from build123d import *

# Parameters (mm, degrees)
SKETCH1_R                 = 2.5
BOSS_EXTRUDE1_DEPTH       = 30
M3X0_5_TAPPED_HOLE1_D     = 2.5
M3X0_5_TAPPED_HOLE1_DEPTH = 7
M3X0_5_TAPPED_HOLE1_TIP   = 0.751075774
M3X0_5_TAPPED_HOLE2_D     = 2.5
M3X0_5_TAPPED_HOLE2_DEPTH = 7
M3X0_5_TAPPED_HOLE2_TIP   = 0.751075774
CHAMFER1_SIZE             = 0.5


with BuildPart() as part:
    # Sketch1 → Boss-Extrude1 (new body)
    with BuildSketch(Plane(origin=(0, 0, 0), x_dir=(1, 0, 0), z_dir=(0, 1, 0))):
        with Locations(Location((0, 0, 0), (0, 0, 270))):
            Circle(SKETCH1_R)
    extrude(amount=BOSS_EXTRUDE1_DEPTH)

    # M3x0.5 Tapped Hole1
    with Locations(Plane(origin=(0, 30, 0), x_dir=(1, 0, 0), z_dir=(0, 1, 0))):
        with Locations((0, 0)):
            Hole(M3X0_5_TAPPED_HOLE1_D / 2, depth=M3X0_5_TAPPED_HOLE1_DEPTH)
            with Locations((0, 0, -(M3X0_5_TAPPED_HOLE1_DEPTH + M3X0_5_TAPPED_HOLE1_TIP / 2))):  # 118° drill point
                Cone(0, M3X0_5_TAPPED_HOLE1_D / 2, M3X0_5_TAPPED_HOLE1_TIP, mode=Mode.SUBTRACT)

    # M3x0.5 Tapped Hole2
    with Locations(Plane(origin=(0, 0, 0), x_dir=(-1, 0, 0), z_dir=(0, -1, 0))):
        with Locations((0, 0)):
            Hole(M3X0_5_TAPPED_HOLE2_D / 2, depth=M3X0_5_TAPPED_HOLE2_DEPTH)
            with Locations((0, 0, -(M3X0_5_TAPPED_HOLE2_DEPTH + M3X0_5_TAPPED_HOLE2_TIP / 2))):  # 118° drill point
                Cone(0, M3X0_5_TAPPED_HOLE2_D / 2, M3X0_5_TAPPED_HOLE2_TIP, mode=Mode.SUBTRACT)

    # Chamfer1
    chamfer1_edges = [part.edges().sort_by_distance(p)[0] for p in [
        (0, 0, -2.5),
        (0, 30, -2.5),
    ]]
    chamfer(chamfer1_edges, length=CHAMFER1_SIZE)


solid = part.part
Read the model definition and answer for the solid it produces. Units are mm, in the model's axes. A direction names the side the tool comes from. Give positions to 0.01 mm unless a question says otherwise; leave off trailing zeros. Write each loop counter-clockwise with the first axis right and the second up, starting at its lowest first coordinate (ties: lowest second). Pieces come first, ordered by that corner, then holes. Notation, with made-up numbers: (81, -6) - (129, -6) arc R18 cw to (129, 16) - close; hole circle Ø5 at (75.5, 10). An arc over 180 degrees is marked (long way). Answer in a Markdown table with one row per item. Add a question column.
Item 1: Section C-C, the plane y = 7.25 is taken. Write down the section's boundary in (x, z), and give its area (3 significant figures).
Item 2: A tool of negligible diameter and unlimited length cuts with its end or side. For faces 4 (the face through (1, 30, 1)), 5 (the face through (0.27, 26.45, 1.22)), 6 (the face through (-0.27, 3.55, 1.22)), from which of +Z, -Z, +X, -X, +Y, -Y can it reach the whole face along a straight path? Write none if from no direction.
Item 3: Section A-A, the plane y = 23.5 is taken. Write down the section's boundary in (x, z), and give its area (3 significant figures).
Item 4: Section B-B, the plane y = 13.5 is taken. Write down the section's boundary in (x, z).
Item 5: Flat-ended cylindrical pins translate along their axes: P1, Ø2, axis at x = 0, z = 0, coming from the -Y side; P2, Ø2, axis at x = -1.5, y = 26.5, coming from the -Z side. Find the tip coordinate at first contact, or state that the pin passes through.
Item 6: Determine the mould class of faces 1 (the face through (-0.05, 22.38, 0.21)), 2 (the face through (-2.44, 14.8, -0.54)), 3 (the face through (1, 0, 1)) for opening direction Z: pulls with the +Z half, pulls with the -Z half, needs draft (parallel to the pull), parting line crosses it, or undercut.
Item 7: Find the intervals of material crossed by L1, parallel to X at y = 3.5, z = 0.15; L2, parallel to Z at x = 0.95, y = 6.25; L3, parallel to Z at x = -1, y = 3.5, in increasing order.
Recorded:
| question | item | result |
|---|---|---|
| 1 | outline | circle Ø5 at (0, 0); hole circle Ø1.67 at (0, 0) |
| 1 | area | 17.5 mm2 |
| 2 | face 4 | +Z, -Z, +X, -X, +Y |
| 2 | face 5 | +Y |
| 2 | face 6 | -Y |
| 3 | outline | circle Ø5 at (0, 0); hole circle Ø2.5 at (0, 0) |
| 3 | area | 14.7 mm2 |
| 4 | outline | circle Ø5 at (0, 0) |
| 5 | P1 | stops at y = 7.15 |
| 5 | P2 | stops at z = -2.45 |
| 6 | face 1 | undercut |
| 6 | face 2 | parting line crosses it |
| 6 | face 3 | needs draft |
| 7 | L1 | x = -2.5 to -1.24, 1.24 to 2.5 |
| 7 | L2 | z = -2.31 to -0.81, 0.81 to 2.31 |
| 7 | L3 | z = -2.29 to -0.75, 0.75 to 2.29 |
